CAD build for the part. Positions are in the model's coordinates, mm. A direction names the side the tool comes from. Give positions to 0.01 mm unless a question says otherwise; leave off trailing zeros. Write each loop counter-clockwise with the first axis right and the second up, starting at its lowest first coordinate (ties: lowest second). Pieces come first, ordered by that corner, then holes. Notation, with made-up numbers: (-29, -15) - (-1, -15) arc R29 ccw to (-1, 9) - close; hole circle Ø9 at (67.5, 10). An arc over 180 degrees is marked (long way). Put each result on its own line as item: value. Start each with the question number.
1. Mould opens along X. For faces 4 (the cylindrical face through (4.012, 23.34, -11.177)), 5 (the flat face through (10.932, 23.134, -10.794)) say: +X half, -X half, draft (parallel to the pull), parting line (faces both ways), or undercut.
2. Cut at C-C on x = 12. List the corners of the cut face in (y, z) (1 decimal).
3. Cut at A-A on x = 24. List the corners of the cut face in (y, z) (1 decimal).
4. Drop flat-ended pins along their axis: pin 1 (5 mm diameter, centred on x = 21, z = -14, fed in from +Y); pin 2 (6 mm diameter, centred on x = 17.5, z = -6, fed in from -Y); pin 3 (4 mm diameter, centred on x = 7.5, z = -7, fed in from -Y); pin 4 (4.5 mm diameter, centred on x = 10, y = 4.5, fed in from -Z). Give the stop position or say it passes through.
5. Tool access for faces 1 (the cylindrical face through (34.13, 23.34, -11.177)), 2 (the flat face through (19, 7, -2)), 3 (the flat face through (27.068, 23.134, -10.794)): list every direction of +Z, -Z, +X, -X, +Y, -Y with a clear straight run to the whole face (end or side of a thin tool).
6. Cut at B-B on y = 8. List the corners of the cut face in (x, z), and give its area (3 significant figures).
7. Cut at D-D on y = 16.5. List the corners of the cut face in (x, z).
8. Wall check: line 1 (Z direction, x = 28, y = 18); line 2 (Z direction, x = 32, y = 8.5); line 3 (Y direction, x = 24, z = -5.75). Give the ranges that are in metal, low to high.
Autodesk Inventor part; units mm, degrees
ref_plane "作業平面1" through (0, -49.7818, -69.441) normal (1, 0, 0) x (0, 0.7071068, -0.7071068)
ref_plane "YZ Plane" through (0, 0, 0) normal (1, 0, 0) x (0, 1, 0)
ref_plane "XZ Plane" through (0, 0, 0) normal (0, 1, 0) x (-1, 0, 0)
sketch "スケッチ1" plane through (0, 0, 0) normal (1, 0, 0) x (0, 1, 0)
  line L0 (0, 0) -> (18, 0)
  line L1 (18, 0) -> (18, -2)
  line L2 (18, -2) -> (0, -2)
  line L3 (0, -2) -> (0, 0)
  line L4 (18, 0) -> (39.2132, -21.2132)
  line L5 (39.2132, -21.2132) -> (37.799, -22.6274)
  line L6 (37.799, -22.6274) -> (17.1716, -2)
  dimension "d0" = 2
  dimension "d1" = 18
  dimension "d4" = 30
  dimension "d5" = 135
  dimension "d6" = 2
extrude "押し出し1" add sketch "スケッチ1" along normal blind 38
sketch "スケッチ2" plane through (38, 0, 0) normal (1, 0, 0) x (0, 0, -1)
  line L0 (13.2259, 26.2762) -> (6.4645, 24.4645)
  line L1 (2, 0) -> (2, 17.1716)
  line L2 (2, 17.1716) -> (22.6274, 37.799)
  line L3 (22.6274, 37.799) -> (21.2132, 39.2132)
  line L4 (21.2132, 39.2132) -> (0, 18)
  line L5 (0, 18) -> (0, 0)
  line L6 (0, 0) -> (2, 0)
  point P0 (10.3282, 25.4997)
extrude "押し出し2" cut sketch "スケッチ2" against normal through all contours L0 L4 L3 L2
sketch "スケッチ3" plane through (38, 0, 0) normal (1, 0, 0) x (0, 0, -1)
  line L0 (0, -0.1838) -> (49.5981, -49.7818)
  line L1 (49.5981, -49.7818) -> (50.9877, -48.3922)
  line L2 (50.9877, -48.3922) -> (50.3051, -40.5894)
  line L3 (50.3051, -40.5894) -> (38.2775, -28.5617)
  line L4 (38.2775, -28.5617) -> (34.3952, -14.0729)
  line L5 (34.3952, -14.0729) -> (39.6985, -8.7696)
  line L6 (25.2028, 5.7261) -> (39.6985, -8.7696)
  line L7 (25.2028, 9.9688) -> (25.2468, 10.0127)
  line L8 (25.2468, 14.2554) -> (13.2259, 26.2762)
  line L9 (13.2259, 26.2762) -> (6.4645, 24.4645)
  line L10 (6.4645, 24.4645) -> (0, 18)
  circle A0 centre (45.0018, -38.8216) radius 0.8
  circle A1 centre (48.5373, -42.3571) radius 0.8
  line L11 (25.2886, 2.8119) -> (28.6525, -0.552)
  arc A2 (29.0919, -1.6127) -> (28.6525, -0.552) centre (27.5919, -1.6127) ccw
  line L12 (29.0919, -1.6127) -> (29.0919, -20.7046)
  arc A3 (26.5312, -21.7652) -> (29.0919, -20.7046) centre (27.5919, -20.7046) ccw
  line L13 (26.5312, -21.7652) -> (23.1673, -18.4013)
  arc A4 (22.7279, -17.3406) -> (23.1673, -18.4013) centre (24.2279, -17.3406) ccw
  line L14 (22.7279, -17.3406) -> (22.7279, 1.7513)
  arc A5 (25.2886, 2.8119) -> (22.7279, 1.7513) centre (24.2279, 1.7513) ccw
  line L15 (13.8033, -9.0373) -> (10.4393, -5.6734)
  arc A6 (10, -4.6127) -> (10.4393, -5.6734) centre (11.5, -4.6127) ccw
  line L16 (10, -4.6127) -> (10, 14.4792)
  arc A7 (12.5607, 15.5398) -> (10, 14.4792) centre (11.5, 14.4792) ccw
  line L17 (12.5607, 15.5398) -> (15.9246, 12.1759)
  arc A8 (16.364, 11.1152) -> (15.9246, 12.1759) centre (14.864, 11.1152) ccw
  line L18 (16.364, 11.1152) -> (16.364, -7.9767)
  arc A9 (13.8033, -9.0373) -> (16.364, -7.9767) centre (14.864, -7.9767) ccw
  line L19 (2, 0) -> (2, 17.1716)
  line L20 (2, 14.3431) -> (13.5795, 25.9226)
  line L21 (16.4919, 23.0102) -> (8.535, 20.8782)
  line L22 (6.4645, 24.4645) -> (0, 18)
  line L23 (2, 17.1716) -> (10.3282, 25.4997)
  circle A10 centre (11.8117, 23.8267) radius 0.8
  circle A11 centre (2.8284, 18) radius 0.8
  circle A12 centre (6.4645, 21.636) radius 0.8
  arc A13 (25.2028, 9.9688) -> (25.2028, 5.7261) centre (27.3241, 7.8475) ccw
  circle A14 centre (16.7615, 19.9122) radius 0.8
  line L24 (0, 18) -> (0, -0.1838)
  arc A15 (25.2468, 10.0127) -> (25.2468, 14.2554) centre (23.1254, 12.1341) ccw
  circle A16 centre (20.297, 16.3767) radius 0.8
  point P0 (0, 0)
  dimension "d9" = 4
  dimension "d10" = 4
ref_plane "作業平面1" through (0, -49.7818, -69.441) normal (1, 0, 0) x (0, 0.7071068, -0.7071068)
extrude "押し出し3" add sketch "スケッチ3" against normal up to surface (38 mm away) contours L9 L8 L20 A10 L19 L23 A11 A12 | A12 L23 | L8 L21 L20 A10 | A10 L20 | L20 A10 | A11 L23 picked at (6.7643, 21.5956) picked at (2.746, 17.7464)
sketch "スケッチ4" plane through (38, 0, 0) normal (1, 0, 0) x (0, 0, -1)
  circle A0 centre (2.8284, 18) radius 0.8
  circle A1 centre (6.4645, 21.636) radius 0.8
  circle A2 centre (11.8117, 23.8267) radius 0.8
  line L0 (6.4645, 24.4645) -> (0, 18)
  line L1 (13.2259, 26.2762) -> (6.4645, 24.4645)
  line L2 (11.8117, 23.8267) -> (11.2941, 25.7586)
  point P0 (0, 0)
  dimension "d13" = 1.6
  dimension "d14" = 2
  dimension "d15" = 2
  dimension "d16" = 2
  dimension "d17" = 2
extrude "押し出し4" cut sketch "スケッチ4" against normal through all
sketch "スケッチ5" plane through (0, 18, 0) normal (0, 0.7071068, 0.7071068) x (1, 0, 0)
  line L0 (19, 8.3282) -> (1.5, 17.1212)
  line L1 (36.5, 17.1212) -> (19, 8.3282)
  line L2 (38, 15.2043) -> (0, 15.2043)
  line L3 (3.0877, 15.2043) -> (19, 7.209)
  line L4 (38, 15.2043) -> (0, 15.2043)
  line L5 (34.9123, 15.2043) -> (19, 7.209)
  point P0 (0, -12.7279)
  dimension "d20" = 1
extrude "押し出し5" cut sketch "スケッチ5" against normal through all
equation "\"d15\" = d14"
properties part number "upper"
Report:
1. face 4: draft
1. face 5: undercut
2. outline: (0, -2) - (14.3, -2) - (20.9, -8.5) - (21.7, -11.5) - (24.9, -8.2) - (24.5, -6.5) - (18, 0) - (0, 0) - close; hole circle Ø1.6 at (18, -2.8); hole circle Ø1.6 at (21.6, -6.5)
3. outline: (0, -2) - (14.3, -2) - (20.9, -8.5) - (21.4, -10.4) - (24.6, -7.1) - (24.5, -6.5) - (18, 0) - (0, 0) - close; hole circle Ø1.6 at (18, -2.8); hole circle Ø1.6 at (21.6, -6.5)
4. pin 1: passes through
4. pin 2: stops at y = 15.34
4. pin 3: stops at y = 17.34
4. pin 4: stops at z = -2
5. face 1: +X, -X
5. face 2: -Z, +X, -X, -Y
5. face 3: -Z, +Y
6. outline: (0, -2) - (38, -2) - (38, 0) - (0, 0) - close
6. area: 76.0 mm²
7. outline: (0, -4.16) - (38, -4.16) - (38, 0) - (0, 0) - close
8. line 1: z = -5.66 to -3.63, -2.03 to 0
8. line 2: z = -2 to 0
8. line 3: y = 18.09 to 21.28, 22 to 23.75
